The listing builds one solid part. Answer for the finished solid, in the listing's coordinates (mm). Give positions to 0.01 mm unless a question says otherwise; leave off trailing zeros. Write each loop counter-clockwise with the first axis right and the second up, starting at its lowest first coordinate (ties: lowest second). Pieces come first, ordered by that corner, then holes. Notation, with made-up numbers: (-15.75, 32.25) - (-10.75, 32.25) arc R22 ccw to (-10.75, 50.25) - close; hole circle Ø2 at (13, 50.25). An arc over 180 degrees is marked (long way). Return JSON: item names as keys, results as strings.
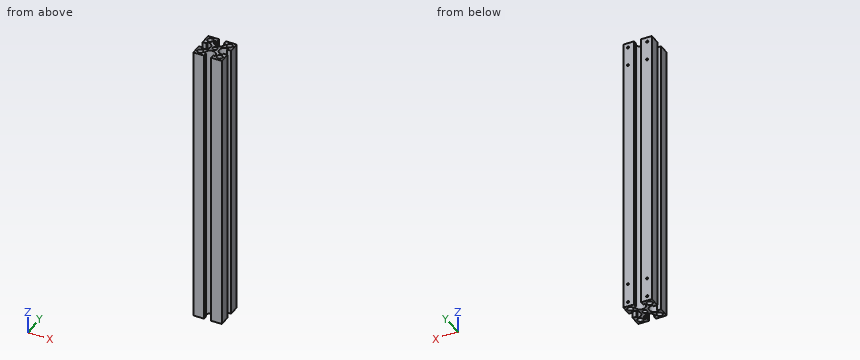
from build123d import *

# Parameters (mm, degrees)
SKETCH_1_W           = 40
SKETCH_1_H           = 40
EXTRUDE_1_DEPTH      = 400
SKETCH_2_R           = 3.25
SKETCH_2_R_2         = 4
CUT_EXTRUDE_1_DEPTH  = 401
M3X0_5_2_D           = 2.5
M3X0_5_2_DEPTH       = 7.5
M3X0_5_2_CBORE_D     = 3
M3X0_5_2_CBORE_DEPTH = 6
M3X0_5_2_TIP         = 0.751075774


with BuildPart() as part:
    # 草圖1 → 伸長1 (new body)
    with BuildSketch(Plane.XY):
        Rectangle(SKETCH_1_W, SKETCH_1_H)
    extrude(amount=EXTRUDE_1_DEPTH)

    # 草圖2 → 除料-伸長1 (cut, through all)
    with BuildSketch(Plane(origin=(0, 0, 0), x_dir=(-1, 0, 0), z_dir=(0, 0, -1))):
        Circle(SKETCH_2_R)
        with Locations((-13.5, 13.5)):
            Circle(SKETCH_2_R_2)
        with Locations((13.5, 13.5)):
            Circle(SKETCH_2_R_2)
        with Locations((-13.5, -13.5)):
            Circle(SKETCH_2_R_2)
        with Locations((13.5, -13.5)):
            Circle(SKETCH_2_R_2)
        with BuildLine():
            Line((5, 14.5), (7.5, 14.5))
            Line((7.5, 14.5), (7.5, 13.5))
            ThreePointArc((7.5, 13.5), (0, 6), (-7.5, 13.5))
            Line((-7.5, 13.5), (-7.5, 14.5))
            Line((-7.5, 14.5), (-5, 14.5))
            Line((-5, 14.5), (-5, 20))
            Line((-5, 20), (5, 20))
            Line((5, 20), (5, 14.5))
        make_face()
        with BuildLine():
            Line((14.5, -5), (14.5, -7.5))
            Line((14.5, -7.5), (13.5, -7.5))
            ThreePointArc((13.5, -7.5), (6, 0), (13.5, 7.5))
            Line((13.5, 7.5), (14.5, 7.5))
            Line((14.5, 7.5), (14.5, 5))
            Line((14.5, 5), (20, 5))
            Line((20, 5), (20, -5))
            Line((20, -5), (14.5, -5))
        make_face()
        with BuildLine():
            Line((-5, -14.5), (-7.5, -14.5))
            Line((-7.5, -14.5), (-7.5, -13.5))
            ThreePointArc((-7.5, -13.5), (0, -6), (7.5, -13.5))
            Line((7.5, -13.5), (7.5, -14.5))
            Line((7.5, -14.5), (5, -14.5))
            Line((5, -14.5), (5, -20))
            Line((5, -20), (-5, -20))
            Line((-5, -20), (-5, -14.5))
        make_face()
        with BuildLine():
            Line((-14.5, 5), (-14.5, 7.5))
            Line((-14.5, 7.5), (-13.5, 7.5))
            ThreePointArc((-13.5, 7.5), (-6, 0), (-13.5, -7.5))
            Line((-13.5, -7.5), (-14.5, -7.5))
            Line((-14.5, -7.5), (-14.5, -5))
            Line((-14.5, -5), (-20, -5))
            Line((-20, -5), (-20, 5))
            Line((-20, 5), (-14.5, 5))
        make_face()
    extrude(amount=-CUT_EXTRUDE_1_DEPTH, mode=Mode.SUBTRACT)

    # M3x0.5 螺紋孔2
    with Locations(Plane(origin=(0, 20, 0), x_dir=(1, 0, 0), z_dir=(0, 1, 0))):
        with Locations((-13.5, -6.5), (-13.5, -33.5), (-13.5, -393.5), (-13.5, -366.5), (13.5, -366.5), (13.5, -393.5), (13.5, -33.5), (13.5, -6.5)):
            CounterBoreHole(M3X0_5_2_D / 2, M3X0_5_2_CBORE_D / 2, M3X0_5_2_CBORE_DEPTH, depth=M3X0_5_2_DEPTH)
            with Locations((0, 0, -(M3X0_5_2_DEPTH + M3X0_5_2_TIP / 2))):  # 118° drill point
                Cone(0, M3X0_5_2_D / 2, M3X0_5_2_TIP, mode=Mode.SUBTRACT)


solid = part.part
Item 1: A cutting plane is placed at A-A on x = 0. Determine the outline of the cut face in (y, z), then the cut area to 3 significant figures.
Answer below:
{"outline": "(-6, 0) - (-3.25, 0) - (-3.25, 400) - (-6, 400) - close; (3.25, 0) - (6, 0) - (6, 400) - (3.25, 400) - close", "area": "2,200 mm²"}
Item 2: A cutting plane is placed at C-C on z = 318. Give the number of separate pieces and of enclosed holes in the cut face, then the cut area to 3 significant figures.
Answer below:
{"separate pieces": "1", "enclosed holes": "5", "area": "732 mm²"}
Item 3: A flat-ended cylindrical pin translates along its axis: P1, Ø1, axis at x = -2, z = 124, coming from the +Y side. Find the tip coordinate at first contact, or state that the pin passes through.
Answer below:
{"P1": "stops at y = 6.43"}
Item 4: Consider L1, parallel to Z at x = 13.5, y = 18.7; L2, parallel to X at y = 19.4, z = 33.5; L3, parallel to Y at x = -13, z = 106. Determine where each line is inside the solid, lowest interval first.
Answer below:
{"L1": "z = 0 to 5, 8 to 32, 35 to 365, 368 to 392, 395 to 400", "L2": "x = -20 to -15, -12 to -5, 5 to 12, 15 to 20", "L3": "y = -20 to -17.47, -9.53 to -7.48, 7.48 to 9.53, 17.47 to 20"}
